Could you check a few things on this model? Use its own coordinates, in mm. Face numbers are marked on the shaded views. A direction names the side the tool comes from. Give positions to 0.01 mm unless a question says otherwise; leave off trailing zeros. Loops run counter-clockwise (first coordinate to the right, second up) from the corner with the lowest first, then second, coordinate; pieces in that order, holes last. Notation, with made-up numbers: M 86.5,56 L 122.5,56 A23 cw 122.5,75 Z; hole C 22.25,-22 d9. An arc over 180 degrees is marked long. Answer in a Markdown table with one row per item. Add a question column.
1. If we section it at B-B on x = 20.5: List the corners of the cut face in (y, z) for me.
2. I need wall thicknesses on line 1 along X through (y, z) = (15.5, 25); line 2 along Z through (x, y) = (-55, 14); line 3 along Y through (x, z) = (43, 26). Which ranges of each line are inside material? Lowest first, please. Write a range as from..to.
3. If we section it at D-D on y = 10.5: List the corners of the cut face in (x, z) for me, then the cut area to 3 significant figures.
4. Which directions (+Z, -Z, +X, -X, +Y, -Y) give clear straight access to the entire face, cutting with the end or side of a thin tool? Please do the marked faces 4 and 5.
5. Thinking about a two-plate mould opening in X: for the marked faces 1, 2 and 3, which applies, released by +X, released by -X, zero draft, split by the parting line, or undercut?
6. If we section it at A-A on z = 3: List the corners of the cut face in (x, y) for me.
7. If we section it at C-C on z = -17.5: List the corners of the cut face in (x, y) for me, then the cut area to 3 significant figures.
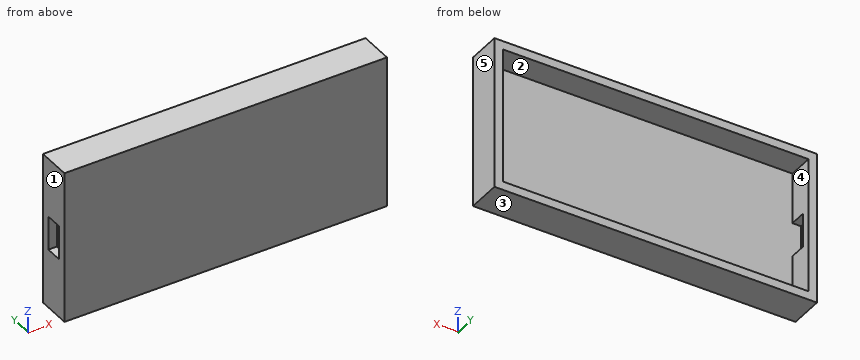
```python
from build123d import *

# Parameters (mm, degrees)
SKETCH3_W           = 190
SKETCH3_H           = 90
SKETCH3_W_2         = 180
SKETCH3_H_2         = 80
BOSS_EXTRUDE2_DEPTH = 20
SKETCH3_4_W         = 15
SKETCH3_4_H         = 10
SKETCH3_4_R         = 7.5
SKETCH3_4_W_2       = 70
SKETCH3_4_H_2       = 35
SKETCH3_4_W_3       = 25
SKETCH3_4_H_3       = 25
BOSS_EXTRUDE3_DEPTH = 5
CUT_EXTRUDE1_DEPTH  = 5


with BuildPart() as part:
    # Sketch3 → Boss-Extrude2 (new body)
    with BuildSketch(Plane(origin=(0, 0, 0), x_dir=(1, 0, 0), z_dir=(0, 1, 0))):
        Rectangle(SKETCH3_W, SKETCH3_H)
        Rectangle(SKETCH3_W_2, SKETCH3_H_2, mode=Mode.SUBTRACT)
    extrude(amount=BOSS_EXTRUDE2_DEPTH)

    # Sketch3_4 → Boss-Extrude3 (add)
    # profile 1 of 5: a face of its own
    with BuildSketch(Plane(origin=(0, 0, 0), x_dir=(1, 0, 0), z_dir=(0, 1, 0))):
        Polygon((-20, 5), (-90, 5), (-90, -40), (65, -40), (65, -15), (90, -15), (90, 40), (-20, 40), align=None)
        with Locations((-12.5, 0)):
            Rectangle(SKETCH3_4_W, SKETCH3_4_H, mode=Mode.SUBTRACT)
        with Locations((75.236819875, 26.883792042)):
            Circle(SKETCH3_4_R, mode=Mode.SUBTRACT)
    # profile 2 of 5: a face of its own
    with BuildSketch(Plane(origin=(0, 0, 0), x_dir=(1, 0, 0), z_dir=(0, 1, 0))):
        with Locations((-12.5, 0)):
            Rectangle(SKETCH3_4_W, SKETCH3_4_H)
    # profile 3 of 5: a face of its own
    with BuildSketch(Plane(origin=(0, 0, 0), x_dir=(1, 0, 0), z_dir=(0, 1, 0))):
        with Locations((-55, 22.5)):
            Rectangle(SKETCH3_4_W_2, SKETCH3_4_H_2)
    # profile 4 of 5: a face of its own
    with BuildSketch(Plane(origin=(0, 0, 0), x_dir=(1, 0, 0), z_dir=(0, 1, 0))):
        with Locations((77.5, -27.5)):
            Rectangle(SKETCH3_4_W_3, SKETCH3_4_H_3)
    # profile 5 of 5: a face of its own
    with BuildSketch(Plane(origin=(0, 0, 0), x_dir=(1, 0, 0), z_dir=(0, 1, 0))):
        with Locations((75.236819875, 26.883792042)):
            Circle(SKETCH3_4_R)
    extrude(amount=BOSS_EXTRUDE3_DEPTH)

    # Sketch4 → Cut-Extrude1 (cut)
    with BuildSketch(Plane.ZY.offset(95)):
        Polygon((-10, 5), (0, 5), (0, 10), (0, 15), (-10, 15), align=None)
        Polygon((0, 10), (0, 5), (10, 5), (10, 15), (0, 15), align=None)
    extrude(amount=-CUT_EXTRUDE1_DEPTH, mode=Mode.SUBTRACT)


solid = part.part
```
Results:
| question | item | result |
|---|---|---|
| 1 | outline | M 0,-45 L 20,-45 L 20,-40 L 5,-40 L 5,40 L 20,40 L 20,45 L 0,45 Z |
| 2 | line 1 | -95..-90, 90..95 |
| 2 | line 2 | -45..-40, 40..45 |
| 2 | line 3 | 0..5 |
| 3 | outline | M -95,-45 L 95,-45 L 95,45 L -95,45 L -95,10 L -90,10 L -90,40 L 90,40 L 90,-40 L -90,-40 L -90,-10 L -95,-10 Z |
| 3 | area | 2,600 mm2 |
| 4 | face 4 | +Y |
| 4 | face 5 | +Z, -Z, +X, +Y, -Y |
| 5 | face 1 | released by -X |
| 5 | face 2 | undercut |
| 5 | face 3 | zero draft |
| 6 | outline | M -95,0 L 95,0 L 95,20 L 90,20 L 90,5 L -95,5 Z; M -95,15 L -90,15 L -90,20 L -95,20 Z |
| 7 | outline | M -95,0 L 95,0 L 95,20 L 90,20 L 90,5 L -90,5 L -90,20 L -95,20 Z |
| 7 | area | 1,100 mm2 |
